Part model, mm, in its own coordinate system. Give positions to 0.01 mm unless a question says otherwise; leave off trailing zeros. Write each loop counter-clockwise with the first axis right and the second up, starting at its lowest first coordinate (ties: lowest second). Pieces come first, ordered by that corner, then holes. Notation, with made-up numbers: (45.25, 84.25) - (65.25, 84.25) arc R25 cw to (65.25, 122.25) - close; hole circle Ø4 at (17.5, 2.5). An arc over 180 degrees is marked (long way). Answer in a Markdown table with one row per item. Add a question column.
1. Band-saw the part on D-D on y = -2.5. Write the cut outline in (x, z), plus the area to 3 significant figures.
2. Pull direction Y, two halves, no side cores. Call faces 1 (the flat face through (12, -5, 0)), 2 (the cylindrical face through (-5, -5, 5)), 3 (the cylindrical face through (28.233, -6.341, 5.577)): released by +Y, released by -Y, zero draft, split by the parting line, or undercut.
3. Band-saw the part on C-C on z = 4. Write the cut outline in (x, y), plus the area to 3 significant figures.
4. Probe line 1 along X through (y, z) = (-2, 4.25); line 2 along Y through (x, z) = (0.5, 9.75); line 3 along X through (y, z) = (-3.5, 9.5). List the from-to ranges inside material, lowest first.
5. Band-saw the part on A-A on y = -5. Write the cut outline in (x, z).
6. Band-saw the part on B-B on x = 23. Write the cut outline in (y, z), plus the area to 3 significant figures.
7. Drop flat-ended pins along their axis: pin 1 Ø2 at (y, z) = (-3.5, 1.5) entering from -X; pin 2 Ø5.5 at (x, y) = (25, -5) entering from -Z; pin 3 Ø1.5 at (y, z) = (-2, 5.5) entering from -X. Give the stop position or say it passes through.
```python
from build123d import *

# Parameters (mm, degrees)
SKETCH1_R           = 5
SKETCH1_W           = 25
SKETCH1_H           = 10
BOSS_EXTRUDE1_DEPTH = 11
SKETCH2_R           = 3.5
CUT_EXTRUDE1_DEPTH  = 11


with BuildPart() as part:
    # Sketch1 → Boss-Extrude1 (new body)
    with BuildSketch(Plane.XY):
        with Locations((25, -5)):
            Circle(SKETCH1_R)
        with Locations((0, -5)):
            Circle(SKETCH1_R)
        with Locations((12.5, -5)):
            Rectangle(SKETCH1_W, SKETCH1_H)
    extrude(amount=BOSS_EXTRUDE1_DEPTH)

    # Sketch2 → Cut-Extrude1 (cut)
    with BuildSketch(Plane.XY.offset(11)):
        with Locations((0.469346028, -5)):
            Circle(SKETCH2_R)
        with Locations((25, -5)):
            Circle(SKETCH2_R)
    extrude(amount=-CUT_EXTRUDE1_DEPTH, mode=Mode.SUBTRACT)


solid = part.part
```
Values:
| question | item | result |
|---|---|---|
| 1 | outline | (-4.33, 0) - (-1.98, 0) - (-1.98, 11) - (-4.33, 11) - close; (2.92, 0) - (22.55, 0) - (22.55, 11) - (2.92, 11) - close; (27.45, 0) - (29.33, 0) - (29.33, 11) - (27.45, 11) - close |
| 1 | area | 262 mm² |
| 2 | face 1 | zero draft |
| 2 | face 2 | split by the parting line |
| 2 | face 3 | undercut |
| 3 | outline | (0, -10) - (25, -10) arc R5 ccw to (25, 0) - (0, 0) arc R5 ccw to start; hole circle Ø7 at (0.47, -5); hole circle Ø7 at (25, -5) |
| 3 | area | 252 mm² |
| 4 | line 1 | x = -4 to -1.33, 2.27 to 23.2, 26.8 to 29 |
| 4 | line 2 | y = -10 to -8.5, -1.5 to 0 |
| 4 | line 3 | x = -4.77 to -2.69, 3.63 to 21.84, 28.16 to 29.77 |
| 5 | outline | (-5, 0) - (-3.03, 0) - (-3.03, 11) - (-5, 11) - close; (3.97, 0) - (21.5, 0) - (21.5, 11) - (3.97, 11) - close; (28.5, 0) - (30, 0) - (30, 11) - (28.5, 11) - close |
| 6 | outline | (-10, 0) - (-7.87, 0) - (-7.87, 11) - (-10, 11) - close; (-2.13, 0) - (0, 0) - (0, 11) - (-2.13, 11) - close |
| 6 | area | 46.8 mm² |
| 7 | pin 1 | stops at x = -4.97 |
| 7 | pin 2 | passes through |
| 7 | pin 3 | stops at x = -4.47 |
